The model under review builds one solid part; all positions refer to its coordinate system, in mm. A direction names the side the tool comes from. Give positions to 0.01 mm unless a question says otherwise; leave off trailing zeros. Loops run counter-clockwise (first coordinate to the right, second up) from the corner with the lowest first, then second, coordinate; pieces in that order, holes last. Notation, with made-up numbers: (28, 17.25) -> (45, 17.25) arc R15 cw to (45, 28.25) -> close; hole circle Ø5 at (13, 89). An arc over 180 degrees is marked (long way). Write each question's results on one line, items separated by ' | '. Start each with the question number.
Q1. Insertion check: pin 1 Ø2 at (x, z) = (44.5, -3.5) entering from -Y; pin 2 Ø1.5 at (x, y) = (-43, -19) entering from -Z; pin 3 Ø5 at (x, z) = (38, -59) entering from +Y. Each pin has a flat end and moves straight along its axis. Give the tip position at first contact, or say it passes through.
Q2. We need section B-B (z = 0). Write out the cut boundary in (x, y), plus the area to 3 significant figures.
Q3. We need section A-A (x = 0). Write out the cut boundary in (y, z).
Q4. We need section C-C (y = -21). Write out the cut boundary in (x, z).
Q5. We need section D-D (x = 21). Write out the cut boundary in (y, z), plus the area to 3 significant figures.
Q6. Machinability: for faces 1 (the face through (-1.382, -54.58, 68.682)), 2 (the face through (-2.17, -7.4, -9.76)), 3 (the face through (-9.764, -19.93, 74.362)), which of the approach directions +Z, -Z, +X, -X, +Y, -Y give a long, thin tool a straight path to every point of the face, cutting with its end or side? Answer none if there is none.
Q7. Wall thickness on L1, parallel to Y at x = 33, z = 32.5; L2, parallel to X at y = -15.5, z = -24; L3, parallel to X at y = -17, z = 21: over which ranges is each line inside the solid? List them lowest first. Write a range as [from, to].
from build123d import *

# Parameters (mm, degrees)
F0_R     = 10
F1_DEPTH = 15
F2_R     = 75
F3_DEPTH = 10
F4_R     = 10.618259
F5_DEPTH = 60


with BuildPart() as f1:
    # F0 (on Front) → F1 (new body)
    with BuildSketch(Plane.XZ):
        Circle(F0_R)
    extrude(amount=F1_DEPTH)

    # F2 (on face) → F3 (join)
    with BuildSketch(Plane.XZ.offset(15)):
        Circle(F2_R)
    extrude(amount=F3_DEPTH)

    # F4 (on face) → F5 (join)
    with BuildSketch(Plane.XZ.offset(25)):
        with Locations((0, 58.153849)):
            Circle(F4_R)
    extrude(amount=F5_DEPTH)


solid = f1.part
Output:
1) pin 1: y = -25 | pin 2: z = -61.97 | pin 3: y = -15
2) outline: (-75, -25) -> (75, -25) -> (75, -15) -> (10, -15) -> (10, 0) -> (-10, 0) -> (-10, -15) -> (-75, -15) -> close | area: 1,800 mm2
3) outline: (-85, 47.54) -> (-25, 47.54) -> (-25, -75) -> (-15, -75) -> (-15, -10) -> (0, -10) -> (0, 10) -> (-15, 10) -> (-15, 75) -> (-25, 75) -> (-25, 68.77) -> (-85, 68.77) -> close
4) outline: circle Ø150 at (0, 0)
5) outline: (-25, -72) -> (-15, -72) -> (-15, 72) -> (-25, 72) -> close | area: 1,440 mm2
6) face 1: -Y | face 2: +Y | face 3: +Y, -Y
7) L1: [-25, -15] | L2: [-71.06, 71.06] | L3: [-72, 72]
